from build123d import *

# Parameters (mm, degrees)
EXTRUDE_1_DEPTH     = 40
SKETCH_4_R          = 11.5
SKETCH_4_R_2        = 1.8
EXTRUDE_3_DEPTH     = 8
CHAMFER_1_SIZE      = 5
CUT_EXTRUDE_4_DEPTH = 32
SKETCH_6_R          = 3
CUT_EXTRUDE_5_DEPTH = 32
SKETCH_7_R          = 3
CUT_EXTRUDE_6_DEPTH = 32


with BuildPart() as part:
    # 草图1 → 凸台-拉伸1 (new body)
    with BuildSketch(Plane.XY):
        with BuildLine():
            Line((0, 47), (0, 83))
            Line((0, 83), (-8, 83))
            Line((-8, 83), (-8, 47))
            ThreePointArc((-8, 47), (8.109127035, 8.109127035), (47, -8))
            Line((47, -8), (83, -8))
            Line((83, -8), (83, 0))
            Line((83, 0), (47, 0))
            ThreePointArc((47, 0), (13.765981284, 13.765981284), (0, 47))
        make_face()
    extrude(amount=EXTRUDE_1_DEPTH)

    # 草图4 → 凸台-拉伸3 (add)
    with BuildSketch(Plane(origin=(0, 0, 0), x_dir=(-1, 0, 0), z_dir=(0, 0, -1))):
        with BuildLine():
            Line((6.74011537, -36.43860018), (36.43860018, -6.74011537))
            Line((36.43860018, -6.74011537), (8, 47))
            ThreePointArc((8, 47), (-8.109127035, 8.109127035), (-47, -8))
            Line((-47, -8), (6.74011537, -36.43860018))
        make_face()
        with Locations((6.74011537, -6.74011537)):
            Circle(SKETCH_4_R, mode=Mode.SUBTRACT)
        with Locations((-15.180194847, -6.74011537)):
            Circle(SKETCH_4_R_2, mode=Mode.SUBTRACT)
        with Locations((6.74011537, 15.180194847)):
            Circle(SKETCH_4_R_2, mode=Mode.SUBTRACT)
        with Locations((6.74011537, -28.660425587)):
            Circle(SKETCH_4_R_2, mode=Mode.SUBTRACT)
        with Locations((28.660425587, -6.74011537)):
            Circle(SKETCH_4_R_2, mode=Mode.SUBTRACT)
    extrude(amount=-EXTRUDE_3_DEPTH)

    # 倒角1
    # the kernel refuses this chamfer: 5 mm, written as the material it adds along each edge
    with BuildSketch(Plane(origin=(47, 47, 8), x_dir=(-0.9727737558517583, 0.23175681203810172, 0), z_dir=(0.23175681203810172, 0.9727737558517583, 0))) as chamfer_1_piece_1_section:
        Polygon((55, CHAMFER_1_SIZE), (55 + CHAMFER_1_SIZE, 0), (55, 0), align=None)
    chamfer_1_piece_1 = revolve(axis=Axis((47, 47, 8), (0, 0, 1)), revolution_arc=116.801049414, mode=Mode.PRIVATE)
    chamfer_1_piece_1 = split(chamfer_1_piece_1, bisect_by=Plane(origin=(21.227823302, -21.638315136, 10.426045108), z_dir=(-0.46773292368325514, 0.8838698502057383, 0)), keep=Keep.TOP, mode=Mode.PRIVATE)
    chamfer_1_piece_1 = split(chamfer_1_piece_1, bisect_by=Plane(origin=(-21.638315136, 21.227823302, 10.426045108), z_dir=(0.8838698502057382, -0.46773292368325536, 0)), keep=Keep.TOP, mode=Mode.PRIVATE)
    add(chamfer_1_piece_1)

    # 草图5 → 切除-拉伸4 (cut)
    with BuildSketch(Plane.XY.offset(40)):
        Polygon((-7.447222151, 23.665476221), (-6.033008589, 25.079689783), (25.079689783, -6.033008589), (23.665476221, -7.447222151), (19.271084521, -11.841613851), (-11.841613851, 19.271084521), align=None)
    extrude(amount=-CUT_EXTRUDE_4_DEPTH, mode=Mode.SUBTRACT)

    # 草图6 → 切除-拉伸5 (cut)
    with BuildSketch(Plane.XZ.offset(8)):
        with Locations(Location((75, 8, 0), (0, 0, 270))):
            Circle(SKETCH_6_R)
        with Locations(Location((75, 32, 0), (0, 0, 270))):
            Circle(SKETCH_6_R)
    extrude(amount=-CUT_EXTRUDE_5_DEPTH, mode=Mode.SUBTRACT)

    # 草图7 → 切除-拉伸6 (cut)
    with BuildSketch(Plane.ZY.offset(8)):
        with Locations((8, 75)):
            Circle(SKETCH_7_R)
        with Locations((32, 75)):
            Circle(SKETCH_7_R)
    extrude(amount=-CUT_EXTRUDE_6_DEPTH, mode=Mode.SUBTRACT)


solid = part.part
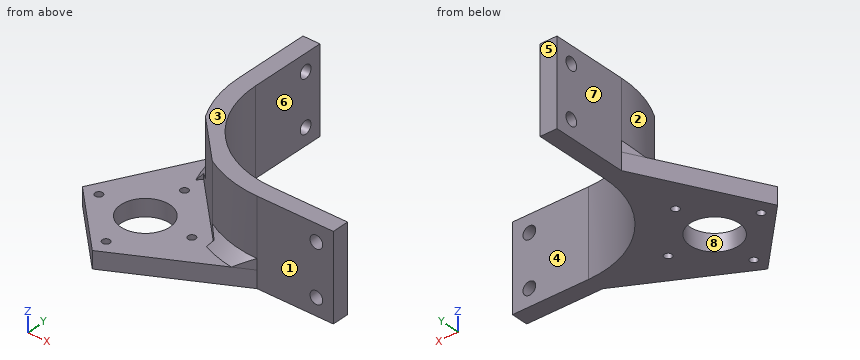
Here's how the part is built. I have some questions about the finished solid (model axes, mm). Face numbers are marked on the shaded views. A direction names the side the tool comes from. Coordinates: 2 decimals unless noted, no trailing zeros. Write each loop counter-clockwise with the first axis right and the second up, starting at its lowest first coordinate (ties: lowest second). Pieces come first, ordered by that corner, then holes.
Item 1: I want a section at D-D on z = 2.5. Write out the boundary of the cut face in (x, y), and give its area (3 significant figures).
Item 2: If we mould it in two halves opening along X, with no side actions, what happens to the marked faces 6, 7 and 8? For each: +X half, -X half, draft (parallel to the pull), parting line (faces both ways), or undercut.
Item 3: Will these pins go through, and if not, where does the flat tip stop? pin 1 (3 mm diameter, centred on x = -6.74, y = -28.66, fed in from -Z); pin 2 (5 mm diameter, centred on x = 23.5, z = 9.5, fed in from -Y); pin 3 (1.5 mm diameter, centred on x = 18.5, z = 7, fed in from +Y); pin 4 (6 mm diameter, centred on x = 65, z = 33, fed in from +Y).
Item 4: I want a section at A-A on z = 32. Write out the boundary of the cut face in (x, y), and give its area (3 significant figures).
Item 5: If I drill on line 1 (Z direction, x = 9, y = 5.5); line 2 (Y direction, x = -3.25, z = 32); line 3 (X direction, y = 49.5, z = 13), over which ranges is the centre line in solid material (lowest first)?
Item 6: I want a section at B-B on y = 75. Write out the boundary of the cut face in (x, z), and give its area (3 significant figures).
Item 7: On a 3-axis mill with a long thin cutter (end or side, diameter ignored), from which of +Z, -Z, +X, -X, +Y, -Y can I reach the whole of each face in a straight line? I mean the marked faces 1, 2, 3, 4 and 5. Say none if no direction works.
Findings below:
1. outline: (-36.44, -6.74) - (-6.74, -36.44) - (47, -8) - (83, -8) - (83, 0) - (47, 0) arc R47 cw to (0, 47) - (0, 83) - (-8, 83) - (-8, 47) - close; hole circle Ø3.6 at (-28.66, -6.74); hole circle Ø23 at (-6.74, -6.74); hole circle Ø3.6 at (-6.74, -28.66); hole circle Ø3.6 at (-6.74, 15.18); hole circle Ø3.6 at (15.18, -6.74)
1. area: 3,380 mm2
2. face 6: +X half
2. face 7: -X half
2. face 8: undercut
3. pin 1: passes through
3. pin 2: stops at y = -21.49
3. pin 3: stops at y = 10.21
3. pin 4: stops at y = 0
4. outline: (-8, 47) arc R55 ccw to (-0.87, 19.92) - (19.92, -0.87) arc R55 ccw to (47, -8) - (72, -8) - (72, 0) - (47, 0) arc R47 cw to (0, 47) - (0, 72) - (-8, 72) - close; (-8, 78) - (0, 78) - (0, 83) - (-8, 83) - close; (78, -8) - (83, -8) - (83, 0) - (78, 0) - close
4. area: 1,080 mm2
5. line 1: z = 0 to 8
5. line 2: y = 24.64 to 72, 78 to 83
5. line 3: x = -8 to 0
6. outline: (-8, 0) - (0, 0) - (0, 5) - (-8, 5) - close; (-8, 11) - (0, 11) - (0, 29) - (-8, 29) - close; (-8, 35) - (0, 35) - (0, 40) - (-8, 40) - close
6. area: 224 mm2
7. face 1: +Z, -Z, +X, -Y
7. face 2: +Z, -X, -Y
7. face 3: +Z, +X, -X, +Y, -Y
7. face 4: +Z, -Z, +X, +Y
7. face 5: +Z, -Z, +X, -X, +Y
